Autodesk Inventor part; units mm, degrees
ref_plane "YZ Plane" through (0, 0, 0) normal (1, 0, 0) x (0, 1, 0)
ref_plane "XZ Plane" through (0, 0, 0) normal (0, 1, 0) x (-1, 0, 0)
ref_plane "XY Plane" through (0, 0, 0) normal (0, 0, 1) x (1, 0, 0)
sketch "Bottom" plane through (0, 0, 0) normal (0, 0, 1) x (1, 0, 0)
  line L0 (0, 0) -> (88.9, 0)
  line L1 (88.9, 0) -> (88.9, -3.0988)
  line L2 (88.9, -3.0988) -> (0, -3.0988)
  line L3 (0, -3.0988) -> (0, 0)
  line L4 (44.45, -3.0988) -> (44.45, 0)
  line L5 (44.45, 0) -> (90.932, 0)
  line L6 (44.45, 0) -> (90.932, 0)
  line L7 (90.932, 0) -> (90.932, -3.0988)
  line L8 (90.932, -3.0988) -> (44.45, -3.0988)
  line L9 (44.45, -3.0988) -> (44.45, 0)
  line L10 (44.45, 0) -> (-2.032, 0)
  line L11 (-2.032, 0) -> (-2.032, -3.0988)
  line L12 (-2.032, -3.0988) -> (44.45, -3.0988)
  line L13 (44.45, -3.0988) -> (44.45, 0)
  dimension "d0" = 88.9
  dimension "d1" = 3.0988
  dimension "d3" = 46.482
  dimension "d4" = 46.482
revolve "Bottom Base" add sketch "Bottom" angle 360 about axis through (44.45, -3.0988, 0) along (0, 1, 0)
sketch "Outer Wall Circles" plane through (44.45, 0, 0) normal (0, 1, 0) x (1, 0, 0)
  circle A0 centre (0, 0) radius 44.45
  circle A1 centre (0, 0) radius 45.72
  point P0 (-44.45, 0)
  dimension "d6" = 88.9
  dimension "d77" = 91.44
extrude "Outer Wall Extr" add sketch "Outer Wall Circles" along normal blind 17.78
sketch "Mount Square" plane through (44.45, -3.0988, 0) normal (0, -1, 0) x (1, 0, 0)
  circle A0 centre (0, 0) radius 46.482
  line L0 (43.307, -46.482) -> (-43.307, -46.482)
  line L1 (-46.482, -43.307) -> (-46.482, 43.307)
  line L2 (-43.307, 46.482) -> (43.307, 46.482)
  line L3 (46.482, 43.307) -> (46.482, -43.307)
  line L4 (46.482, -46.482) -> (-46.482, 46.482) construction
  line L5 (-46.482, -46.482) -> (46.482, 46.482) construction
  arc A1 (-46.482, -43.307) -> (-43.307, -46.482) centre (-43.307, -43.307) ccw
  arc A2 (43.307, -46.482) -> (46.482, -43.307) centre (43.307, -43.307) ccw
  arc A3 (46.482, 43.307) -> (43.307, 46.482) centre (43.307, 43.307) ccw
  arc A4 (-43.307, 46.482) -> (-46.482, 43.307) centre (-43.307, 43.307) ccw
  point P0 (-44.45, 0)
  dimension "d30" = 3.175
extrude "Base Mount" add sketch "Mount Square" against normal blind 3.0988 contours L3 A2 L0 A0 | A0 L2 A3 L3 | A0 L1 A4 L2 | L0 A1 L1 A0
sketch "Silicon Circles" plane through (1.143, -3.0988, 46.482) normal (0, -1, 0) x (1, 0, 0)
  line L0 (89.789, -3.175) -> (89.789, -89.789)
  circle A0 centre (43.1405, -46.482) radius 44.45
  circle A1 centre (43.1405, -46.482) radius 43.18
  point P0 (-1.143, -46.482)
  dimension "d37" = 88.9
  dimension "d38" = 86.36
extrude "Silicon Hole" cut sketch "Silicon Circles" against normal blind 1.0414
sketch "HX711-MCU Design" plane through (44.45, 0, 0) normal (0, 1, 0) x (1, 0, 0)
  line L0 (0, 0) -> (-44.45, 0) construction
  line L1 (-23.3172, -8.1296) -> (-30.9372, -8.1296)
  line L2 (-30.9372, -8.1296) -> (-30.9372, -25.9096)
  line L3 (-30.9372, -25.9096) -> (-23.3172, -25.9096)
  line L4 (-23.3172, -25.9096) -> (-23.3172, -8.1296)
  dimension "d57" = 7.62
  dimension "d58" = 17.78
extrude "HX711 - MCU Hole" cut sketch "HX711-MCU Design" against normal blind 3.1242
sketch "hx711 mount" plane through (44.45, 0, 0) normal (0, 1, 0) x (1, 0, 0)
  line L0 (20.11, -38.7522) -> (-20.11, -38.7522)
  line L1 (-20.11, -38.7522) -> (-20.11, -32.6906)
  line L2 (-20.11, -10.3514) -> (20.11, -10.3514)
  line L3 (20.11, -10.3514) -> (20.11, -16.413)
  line L4 (17.765, -37.0963) -> (-17.765, -12.0073) construction
  line L5 (-17.765, -37.0963) -> (17.765, -12.0073) construction
  line L6 (17.765, -37.0963) -> (-17.765, -37.0963)
  line L7 (-17.765, -37.0963) -> (-17.765, -32.6906)
  line L8 (-17.765, -12.0073) -> (17.765, -12.0073)
  line L9 (17.765, -12.0073) -> (17.765, -16.413)
  line L10 (17.765, -37.0963) -> (-17.765, -12.0073) construction
  line L11 (-17.765, -37.0963) -> (-11.5259, -32.6906) construction
  line L12 (0, -24.5518) -> (17.765, -24.5518) construction
  line L13 (-17.765, -32.6906) -> (-20.11, -32.6906)
  line L14 (-11.5259, -32.6906) -> (17.765, -12.0073) construction
  line L15 (-20.11, -16.413) -> (-17.765, -16.413)
  line L16 (17.765, -32.6906) -> (20.11, -32.6906)
  line L17 (17.765, -16.413) -> (20.11, -16.413)
  line L18 (-17.765, -12.0073) -> (17.765, -12.0073)
  line L19 (17.765, -12.0073) -> (17.765, -16.413)
  line L20 (17.765, -37.0963) -> (-17.765, -37.0963)
  line L21 (-17.765, -37.0963) -> (-17.765, -32.6906)
  line L22 (-20.11, -38.7522) -> (20.11, -38.7522)
  line L23 (20.11, -38.7522) -> (20.11, -32.6906)
  line L24 (20.11, -10.3514) -> (-20.11, -10.3514)
  line L25 (-20.11, -10.3514) -> (-20.11, -16.413)
  line L26 (-17.765, -16.413) -> (-17.765, -12.0073)
  line L27 (-20.11, -16.413) -> (-20.11, -10.3514)
  line L28 (17.765, -32.6906) -> (17.765, -37.0963)
  line L29 (17.765, -32.6906) -> (17.765, -37.0963)
  line L30 (20.11, -32.6906) -> (20.11, -38.7522)
  line L31 (20.11, -16.413) -> (20.11, -10.3514)
  line L32 (-20.11, -32.6906) -> (-20.11, -38.7522)
  line L33 (-17.765, -16.413) -> (-17.765, -12.0073)
  point P0 (-44.45, 0)
  point P1 (-17.765, -32.6906)
sketch "Bottom Circles" plane through (44.45, 0, 0) normal (0, 1, 0) x (1, 0, 0)
  line L0 (-16.2451, -6.4091) -> (-16.2451, 6.2909) construction
  line L1 (-22.9507, -0.0591) -> (-16.2451, -0.0591) construction
  line L2 (-22.9507, -0.0591) -> (-18.3787, -0.0591) construction
  circle A0 centre (-20.6647, -0.0591) radius 2.286
  line L3 (-33.3647, -0.0591) -> (-22.9507, -0.0591) construction
  line L4 (-33.3647, -0.0591) -> (-40.0703, -0.0591) construction
  line L5 (-40.0703, 6.2909) -> (-40.0703, -6.4091) construction
  line L6 (-16.2451, -6.4091) -> (-40.0703, -6.4091) construction
  line L7 (-40.0703, -6.4091) -> (-40.0703, 6.2909) construction
  line L8 (-40.0703, 6.2909) -> (-16.2451, 6.2909) construction
  line L9 (-16.2451, 6.2909) -> (-16.2451, -6.4091) construction
  line L10 (-28.1577, -0.0591) -> (-28.1577, -6.4091) construction
  line L11 (-40.0703, -6.4091) -> (-16.2451, -6.4091) construction
  circle A1 centre (-35.6507, -0.0591) radius 2.286
  line L12 (0, 0) -> (0, 6.2909) construction
  line L13 (0, 0) -> (-45.3601, 45.3601) construction
  line L14 (0, 0) -> (64.1489, 0) construction
  circle A2 centre (-39.6699, 39.6699) radius 3.15
  circle A3 centre (39.6699, 39.6699) radius 3.15
  line L15 (0, 0) -> (6.017, 0) construction
  circle A4 centre (-39.6699, -39.6699) radius 3.15
  circle A5 centre (39.6699, -39.6699) radius 3.15
  point P0 (-44.45, 0)
  dimension "d103" = 4.572
  dimension "d104" = 10.414
  dimension "d105" = 2.1336
  dimension "d106" = 2.1336
  dimension "d113" = 135
  dimension "d114" = 6.3
extrude "Bottom Holes" cut sketch "Bottom Circles" against normal blind 4 contours A0 | A1
sketch "Top Shadow" plane through (44.45, 0, 0) normal (0, 1, 0) x (1, 0, 0)
  line L0 (27.4022, -6.3354) -> (27.4022, 6.3646) construction
  circle A0 centre (34.8952, 0.0146) radius 2.794 construction
  circle A1 centre (19.9092, 0.0146) radius 2.794 construction
  line L1 (22.7032, 0.0146) -> (32.1012, 0.0146) construction
  line L2 (14.7022, -6.3354) -> (40.1022, -6.3354) construction
  line L3 (40.1022, -6.3354) -> (40.1022, 6.3646) construction
  line L4 (40.1022, 6.3646) -> (14.7022, 6.3646) construction
  line L5 (14.7022, 6.3646) -> (14.7022, -6.3354) construction
  line L6 (14.7022, -6.3354) -> (40.1022, 6.3646) construction
  line L7 (40.1022, -6.3354) -> (14.7022, 6.3646) construction
  line L8 (40.065, -6.3646) -> (-40.065, -6.3646) construction
  line L9 (-40.065, -6.3646) -> (-40.065, 6.3646) construction
  line L10 (-40.065, 6.3646) -> (40.065, 6.3646) construction
  line L11 (40.065, 6.3646) -> (40.065, -6.3646) construction
  line L12 (40.065, -6.3646) -> (-40.065, 6.3646) construction
  line L13 (-40.065, -6.3646) -> (40.065, 6.3646) construction
  point P0 (27.4022, 0.0146)
  point P1 (0, 0)
  dimension "d109" = 9.398
extrude "Base to Rail Mount" cut sketch "Bottom Circles" against normal blind 4 contours A2 | A3 | A4 | A5
extrude "hx711 walls" add sketch "hx711 mount" along normal blind 10
properties part number "Bottom Sensor Base v1.3"
Model file for the job. Use its own axes, mm. A direction names the side the tool comes from. Give positions to 0.01 mm unless a question says otherwise; leave off trailing zeros. Order: outer loops, then holes, each group sorted by start corner. A loop starts at its lowest first (then second) coordinate and runs counter-clockwise, first axis right, second up. Notation, with made-up numbers: (63, -11.5) - (102, -11.5) arc R28 ccw to (102, 25.5) - close; hole circle Ø4 at (-23, 53.25). An arc over 180 degrees is marked (long way). One line per item, written item: value.
Item 1: Slice it at A-A (y = 2.75). List the corners of the cut face in (x, z) (3 decimals), then the cut area to 3 significant figures.
Response values:
outline: circle Ø91.44 at (44.45, 0); (24.34, 10.351) - (64.56, 10.351) - (64.56, 16.413) - (62.215, 16.413) - (62.215, 12.007) - (26.685, 12.007) - (26.685, 16.413) - (24.34, 16.413) - close; (24.34, 32.691) - (26.685, 32.691) - (26.685, 37.096) - (62.215, 37.096) - (62.215, 32.691) - (64.56, 32.691) - (64.56, 38.752) - (24.34, 38.752) - close; hole circle Ø88.9 at (44.45, 0)
area: 534 mm2
Item 2: Slice it at C-C (z = -38.5). List the corners of the cut face in (x, y), then the cut area to 3 significant figures.
Response values:
outline: (-2.03, -3.1) - (1.86, -3.1) - (1.86, 0) - (-2.03, 0) - close; (7.7, -3.1) - (22.07, -3.1) - (22.07, -2.06) - (24.73, -2.06) - (24.73, -3.1) - (63.84, -3.1) - (63.84, -2.06) - (66.5, -2.06) - (66.5, -3.1) - (81.2, -3.1) - (81.2, 0) - (69.11, 0) - (69.11, 17.78) - (66.67, 17.78) - (66.67, 0) - (22.23, 0) - (22.23, 17.78) - (19.79, 17.78) - (19.79, 0) - (7.7, 0) - close; (87.04, -3.1) - (90.93, -3.1) - (90.93, 0) - (87.04, 0) - close
area: 333 mm2
Item 3: Slice it at D-D (x = 75.5). List the corners of the cut face in (y, z), then the cut area to 3 significant figures.
Response values:
outline: (-3.1, -46.48) - (0, -46.48) - (0, -33.56) - (17.78, -33.56) - (17.78, -31.81) - (0, -31.81) - (0, 31.81) - (17.78, 31.81) - (17.78, 33.56) - (0, 33.56) - (0, 46.48) - (-3.1, 46.48) - (-3.1, 31.64) - (-2.06, 31.64) - (-2.06, 29.83) - (-3.1, 29.83) - (-3.1, -29.83) - (-2.06, -29.83) - (-2.06, -31.64) - (-3.1, -31.64) - close
area: 347 mm2
Item 4: Two-plate mould, pull along X, no slides. Class faces 4 (the flat face through (21.133, -2, 17)), 5 (the flat face through (44, -3.099, 45)), 6 (the flat face through (90.932, -2, 1)): released by +X, released by -X, zero draft, split by the parting line, or undercut.
Response values:
face 4: undercut
face 5: zero draft
face 6: released by +X
Item 5: Tool access for faces 1 (the flat face through (26, 5, 32.691)), 2 (the cylindrical face through (-0.124, -2.585, 1.954)), 3 (the flat face through (13.513, -2, 17)): list every direction of +Z, -Z, +X, -X, +Y, -Y with a clear straight run to the whole face (end or side of a thin tool).
Response values:
face 1: +Y
face 2: -Y
face 3: +Y, -Y
Item 6: Pin check, flat tips, straight feed: pin 1 Ø1 at (y, z) = (11, 2.5) entering from +X; pin 2 Ø5 at (x, z) = (4.78, 39.67) entering from -Y; pin 3 Ø3 at (x, z) = (65, -17) entering from +Y; pin 4 Ø1 at (y, z) = (2.5, 30.5) entering from +X. Stop position of each tip, or through.
Response values:
pin 1: x = 90.13
pin 2: through
pin 3: y = 0
pin 4: x = 78.95
Item 7: Slice it at B-B (x = 17.5). List the corners of the cut face in (y, z).
Response values:
outline: (-3.1, -46.48) - (0, -46.48) - (0, -36.93) - (17.78, -36.93) - (17.78, -35.35) - (0, -35.35) - (0, 8.13) - (-3.1, 8.13) - (-3.1, -33.87) - (-2.06, -33.87) - (-2.06, -35.47) - (-3.1, -35.47) - close; (-3.1, 25.91) - (0, 25.91) - (0, 35.35) - (17.78, 35.35) - (17.78, 36.93) - (0, 36.93) - (0, 46.48) - (-3.1, 46.48) - (-3.1, 35.47) - (-2.06, 35.47) - (-2.06, 33.87) - (-3.1, 33.87) - close
Item 8: Wall check: line 1 (Z direction, x = 36, y = 8); line 2 (X direction, y = 10.25, z = 0); line 3 (Z direction, x = 46, y = 2.25). Give the ranges that are in metal, low to high.
Response values:
line 1: -44.93 to -43.64, 10.35 to 12.01, 37.1 to 38.75, 43.64 to 44.93
line 2: -1.27 to 0, 88.9 to 90.17
line 3: -45.69 to -44.42, 10.35 to 12.01, 37.1 to 38.75, 44.42 to 45.69
